```python
from build123d import *

# Parameters (mm, degrees)
SKETCH_1_R        = 13
EXTRUDE_477_DEPTH = 14
CHAMFER_1_SIZE    = 2


with BuildPart() as part:
    # 草图1 → Extrude 477 (new body)
    with BuildSketch(Plane.XY):
        Polygon((0, 0), (45, 0), (70, 25), (70, 205), (45, 230), (0, 230), align=None)
        with Locations((35, 35)):
            Circle(SKETCH_1_R, mode=Mode.SUBTRACT)
        with Locations((35, 115)):
            Circle(SKETCH_1_R, mode=Mode.SUBTRACT)
        with Locations((35, 195)):
            Circle(SKETCH_1_R, mode=Mode.SUBTRACT)
    extrude(amount=EXTRUDE_477_DEPTH)

    # 倒角1
    chamfer_1_edges = [part.edges().sort_by_distance(p)[0] for p in [
        (57.5, 12.5, 14),
        (70, 115, 14),
        (57.5, 217.5, 14),
        (22, 35, 0),
        (22, 35, 14),
        (22.5, 230, 14),
        (22, 115, 0),
        (22, 115, 14),
        (22, 195, 0),
        (22, 195, 14),
        (0, 115, 14),
        (22.5, 230, 0),
        (57.5, 217.5, 0),
        (70, 115, 0),
        (22.5, 0, 14),
        (57.5, 12.5, 0),
        (22.5, 0, 0),
        (0, 115, 0),
    ]]
    chamfer(chamfer_1_edges, length=CHAMFER_1_SIZE)


solid = part.part
```
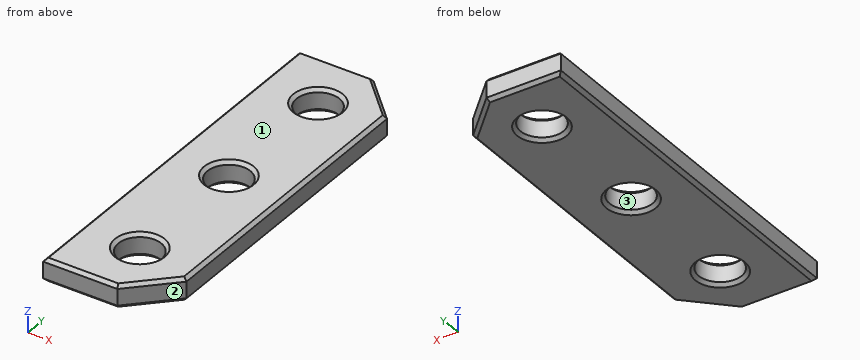
The model under review builds one solid part; all positions refer to its coordinate system, in mm. Face numbers are marked on the shaded views. Coordinates: 2 decimals unless noted, no trailing zeros. Loops run counter-clockwise (first coordinate to the right, second up) from the corner with the lowest first, then second, coordinate; pieces in that order, holes last. Notation, with made-up numbers: (62.5, 2) -> (78.5, 2) arc R6 ccw to (78.5, 9) -> close; hole circle Ø8 at (-22.5, -9.75). An arc over 180 degrees is marked (long way). Answer as CSV lines item,"result".
Item 1: Take a section at A-A, the plane y = 35. State the section outline as (x, z) points, and give its area (3 significant figures).
Results below:
outline,"(0, 2) -> (2, 0) -> (20, 0) -> (22, 2) -> (22, 12) -> (20, 14) -> (2, 14) -> (0, 12) -> close; (48, 2) -> (50, 0) -> (68, 0) -> (70, 2) -> (70, 12) -> (68, 14) -> (50, 14) -> (48, 12) -> close"
area,"600 mm2"
Item 2: Take a section at D-D, the plane x = 52.5. State the section outline as (y, z) points.
Results below:
outline,"(7.5, 2) -> (10.33, 0) -> (219.67, 0) -> (222.5, 2) -> (222.5, 12) -> (219.67, 14) -> (10.33, 14) -> (7.5, 12) -> close"
Item 3: For L1, parallel to Y at x = 34, z = 7.5; L2, parallel to Y at x = 27.5, z = 11.75; L3, parallel to X at y = 189, z = 10.75, list the stretches that pass through material, from the lowest coordinate up.
Results below:
L1,"y = 0 to 22.04, 47.96 to 102.04, 127.96 to 182.04, 207.96 to 230"
L2,"y = 0 to 24.38, 45.62 to 104.38, 125.62 to 184.38, 205.62 to 230"
L3,"x = 0 to 23.47, 46.53 to 70"
Item 4: Insertion check: pin 1 (2 mm diameter, centred on x = 23, y = 139, fed in from -Z); pin 2 (1 mm diameter, centred on x = 51, z = 3.5, fed in from -Y). Each pin has a flat end and moves straight along its axis. Give the tip position at first contact, or say it passes through.
Results below:
pin 1,"stops at z = 0"
pin 2,"stops at y = 5.5"
Item 5: Take a section at B-B, the plane x = 35. Count the separate pieces of the cut face and the enclosed holes in it, and give its area (3 significant figures).
Results below:
separate pieces,"4"
enclosed holes,"0"
area,"2,100 mm2"
Item 6: Draft analysis for pull direction X (two halves, no side actions). For the marked faces 1, 2 and 3, state which applies: +X half, -X half, draft (parallel to the pull), parting line (faces both ways), or undercut.
Results below:
face 1,"draft"
face 2,"+X half"
face 3,"undercut"
Item 7: Take a section at C-C, the plane z = 5.5. State the section outline as (x, y) points.
Results below:
outline,"(0, 0) -> (45, 0) -> (70, 25) -> (70, 205) -> (45, 230) -> (0, 230) -> close; hole circle Ø26 at (35, 35); hole circle Ø26 at (35, 115); hole circle Ø26 at (35, 195)"
